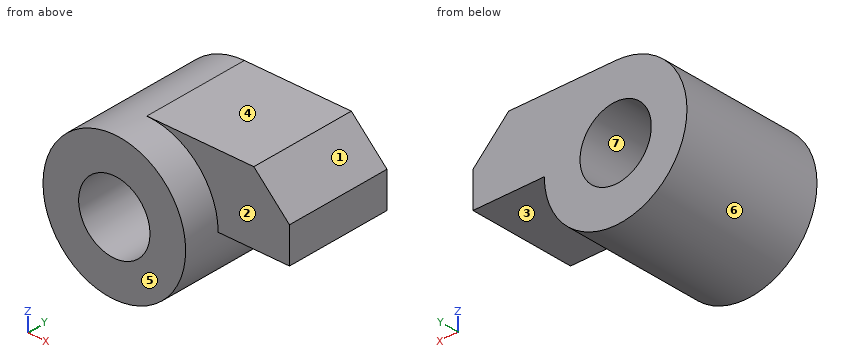
```python
from build123d import *

# Parameters (mm, degrees)
F0_R     = 10
F0_R_2   = 5
F1_DEPTH = 20
F3_DEPTH = 15


with BuildPart() as f1:
    # F0 (on Front) → F1 (new body)
    with BuildSketch(Plane.XZ):
        Circle(F0_R)
        Circle(F0_R_2, mode=Mode.SUBTRACT)
    extrude(amount=-F1_DEPTH)

    # F2 (on face) → F3 (join)
    with BuildSketch(Plane(origin=(0, 20, 0), x_dir=(-1, 0, 0), z_dir=(0, 1, 0))):
        with BuildLine():
            Line((-15, 10), (-20, 5))
            Line((-20, 5), (-20, 0))
            Line((-20, 0), (-10, 0))
            ThreePointArc((-10, 0), (-7.071068, 7.071068), (0, 10))
            Line((0, 10), (-15, 10))
        make_face()
    extrude(amount=-F3_DEPTH)


solid = f1.part
```
Part model, mm, in its own coordinate system. Face numbers are marked on the shaded views. A direction names the side the tool comes from. Round coordinates to 2 decimals unless told otherwise and drop trailing zeros. Loops run counter-clockwise (first coordinate to the right, second up) from the corner with the lowest first, then second, coordinate; pieces in that order, holes last.
1. Slice it at A-A (z = -3.5). Give the cut face in (x, y).
Solutions:
outline: (-9.37, 0) - (-3.57, 0) - (-3.57, 20) - (-9.37, 20) - close; (3.57, 0) - (9.37, 0) - (9.37, 20) - (3.57, 20) - close
2. Slice it at B-B (y = 18.75). Give the cut face in (x, z), and give its area (3 significant figures).
Solutions:
outline: (0, 10) arc R10 ccw (long way) to (10, 0) - (20, 0) - (20, 5) - (15, 10) - close; hole circle Ø10 at (0, 0)
area: 345 mm2
3. Flat gauge pins, fed straight in: pin 1 (3 mm diameter, centred on x = 13.5, y = 9, fed in from -Z); pin 2 (8 mm diameter, centred on y = 5.5, z = 8, fed in from -X); pin 3 (1.5 mm diameter, centred on y = 17, z = 5, fed in from -X); pin 4 (5 mm diameter, centred on x = 12, z = 2.5, fed in from -Y). Where does each tip first touch, or does it go through?
Solutions:
pin 1: stops at z = 0
pin 2: stops at x = -9.17
pin 3: stops at x = -9.05
pin 4: stops at y = 0
4. Two-plate mould, pull along Z, no slides. Class the marked faces 4, 5, 6 and 7: pulls with the +Z half, pulls with the -Z half, needs draft (parallel to the pull), parting line crosses it, or undercut.
Solutions:
face 4: pulls with the +Z half
face 5: needs draft
face 6: parting line crosses it
face 7: undercut
5. Drill centre lines: line 1 along X through (y, z) = (2.25, -0.25); line 2 along Y through (x, z) = (17.25, 4.25); line 3 along X through (y, z) = (12, 1.5). Where is each one in solid material? Low to high.
Solutions:
line 1: x = -10 to -4.99, 4.99 to 10
line 2: y = 5 to 20
line 3: x = -9.89 to -4.77, 4.77 to 20
6. Slice it at D-D (x = 14.25). Give the cut face in (y, z).
Solutions:
outline: (5, 0) - (20, 0) - (20, 10) - (5, 10) - close
7. 3-axis set-ups, long thin cutter, end or side, ignore diameter. For the marked faces 1, 2 and 3: which of +Z, -Z, +X, -X, +Y, -Y reach the whole face in a straight line?
Solutions:
face 1: +Z, +X, +Y, -Y
face 2: +Z, +X, -Y
face 3: -Z, +X, +Y, -Y
